Here's the drawing with two shaded views (mm, measured from the low corner). I have some questions. A direction names the side the tool comes from. Round coordinates to 2 decimals unless told otherwise and drop trailing zeros. Order: outer loops, then holes, each group sorted by start corner. A loop starts at its lowest first (then second) coordinate and runs counter-clockwise, first axis right, second up. Notation, with made-up numbers: (3.25, -14) - (39.25, -14) arc R24 cw to (39.25, 7) - close; hole circle Ø6 at (60, 39). An arc over 180 degrees is marked (long way). Return JSON: item names as keys, results as strings. Group by question number.
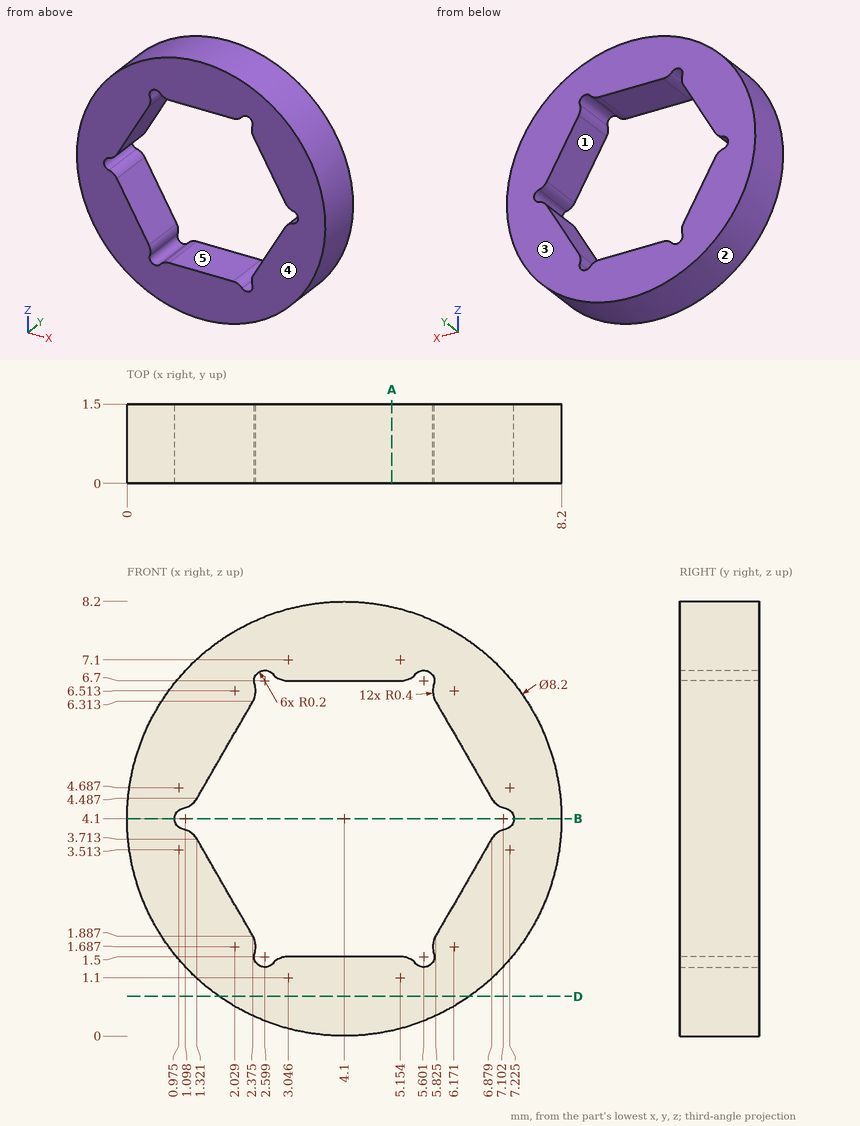
1) I want a section at A-A, the plane x = 5. List the corners of the cut face in (y, z) for me.
2) I want a section at B-B, the plane z = 4.1. List the corners of the cut face in (x, y) for me.
3) I want a section at D-D, the plane z = 0.75. List the corners of the cut face in (x, y) for me.
4) We'd pull the mould along Z, two halves only. Please class the marked faces 1, 2 and 3: +Z half, -Z half, draft (parallel to the pull), parting line (faces both ways), or undercut.
5) Will this pin go through, and if not, where does the flat tip stop? pin 1 (4 mm diameter, centred on x = 4.5, z = 3, fed in from -Y).
6) For the marked faces 4 and 5, which set-ups out of +Z, -Z, +X, -X, +Y, -Y let a thin tool reach every point of the face, with its end or its side?
7) If I drill on line 1 along Z through (x, y) = (4, 1.4); line 2 along X through (y, z) = (0.5, 3); line 3 along Z through (x, y) = (2.75, 0.65), over which ranges is the centre line in solid material (lowest first)? Write a range as from..to.
Outcome:
{
 "1": {"outline": "(0, 0.1) - (1.5, 0.1) - (1.5, 1.5) - (0, 1.5) - close; (0, 6.7) - (1.5, 6.7) - (1.5, 8.1) - (0, 8.1) - close"},
 "2": {"outline": "(0, 0) - (0.9, 0) - (0.9, 1.5) - (0, 1.5) - close; (7.3, 0) - (8.2, 0) - (8.2, 1.5) - (7.3, 1.5) - close"},
 "3": {"outline": "(1.74, 0) - (6.46, 0) - (6.46, 1.5) - (1.74, 1.5) - close"},
 "4": {"face 1": "undercut", "face 2": "parting line", "face 3": "draft"},
 "5": {"pin 1": "y = 0"},
 "6": {"face 4": "+Z, -Z, +X, -X, -Y", "face 5": "+Y, -Y"},
 "7": {"line 1": "0..1.5, 6.7..8.2", "line 2": "0.15..1.73, 6.47..8.05", "line 3": "0.23..1.37, 6.83..7.97"}
}
